Autodesk Inventor part; units mm, degrees
ref_plane "YZ Plane" through (0, 0, 0) normal (1, 0, 0) x (0, 1, 0)
ref_plane "XZ Plane" through (0, 0, 0) normal (0, 1, 0) x (-1, 0, 0)
ref_plane "XY Plane" through (0, 0, 0) normal (0, 0, 1) x (1, 0, 0)
sketch "Sketch1" plane through (0, 0, 0) normal (0, 0, 1) x (1, 0, 0)
  line L0 (0, 0) -> (24, 0)
  line L1 (24, 0) -> (24, 24)
  line L2 (24, 24) -> (0, 24)
  line L3 (0, 24) -> (0, 0)
  dimension "d0" = 24
  dimension "d1" = 24
extrude "Extrusion1" add sketch "Sketch1" along normal blind 15
sketch "Sketch2" plane through (0, 0, 15) normal (0, 0, 1) x (1, 0, 0)
  line L0 (24, 0) -> (24, 24)
  line L1 (24, 24) -> (0, 24)
  line L2 (0, 24) -> (0, 0)
  line L3 (0, 0) -> (24, 0)
  line L4 (2, 22) -> (22, 22)
  line L5 (22, 22) -> (22, 2)
  line L6 (22, 2) -> (2, 2)
  line L7 (2, 2) -> (2, 22)
  dimension "d4" = 2
extrude "Extrusion2" add sketch "Sketch2" along normal blind 2.5
chamfer "Chamfer1" distance 2 angle 45 4 edges at (0, 24, 8.75) (0, 0, 8.75) (24, 0, 8.75) (24, 24, 8.75)
sketch "Sketch3" plane through (0, 0, 0) normal (0, 0, -1) x (-1, 0, 0)
  line L0 (-2, 22) -> (-2, 2)
  line L1 (-2, 2) -> (-22, 2)
  line L2 (-22, 2) -> (-22, 22)
  line L3 (-22, 22) -> (-2, 22)
  point P0 (0, 0)
  point P1 (-12, 16)
  point P2 (-12, 22)
  dimension "d10" = 6
hole "Hole1" at (12, 16, 0) direction (0, 0, 1) diameter 4 depth 24 counterbore diameter 6.5 counterbore depth 10
chamfer "Chamfer2" distance 1 angle 45 8 edges at (12, 0, 0) (23, 1, 0) (24, 12, 0) (23, 23, 0) (12, 24, 0) (0, 12, 0) (1, 23, 0) (1, 1, 0)
thicken "Thicken1" operation add thickness 0.1 both sides no extend neighbours yes toward (1, 0, 0) faces at (22, 15.3333, 16.6667) (15.3333, 2, 16.6667) (2, 8.6667, 16.6667) (8.6667, 22, 15.8333)
chamfer "Chamfer3" distance 1.25 angle 45 1 edges at (12, 14, 10)
properties part number "Idle Side Foot"
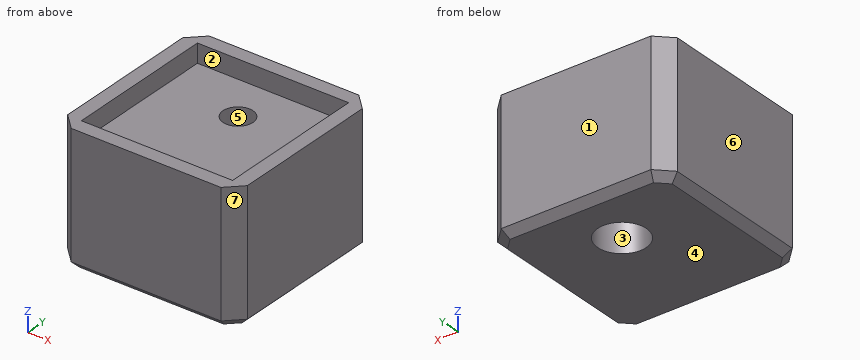
Input: part model. Units: mm. Frame: model coordinates. Face numbers are marked on the shaded views. A direction names the side the tool comes from. Round coordinates to 2 decimals unless told otherwise and drop trailing zeros. Loops run counter-clockwise (first coordinate to the right, second up) from the corner with the lowest first, then second, coordinate; pieces in that order, holes last.
1) Pin query (flat end, axial travel): pin 1 (2 mm diameter, centred on x = 12.5, y = 15.5, fed in from -Z); pin 2 (5 mm diameter, centred on x = 18.5, y = 7.5, fed in from +Z). Return the tip coordinate at first contact, or that it passes through.
Ans:
pin 1: passes through
pin 2: stops at z = 15
2) Set-up query: the marked faces 1, 2 and 3. Return all of +Z, -Z, +X, -X, +Y, -Y with unobstructed straight access to the full face (end or side cutting, diameter ignored); none if empty.
Ans:
face 1: +Z, -Z, +X, -X, +Y
face 2: +Z
face 3: -Z
3) Section query D-D on y = 6.75. Return the cut outline in (x, z).
Ans:
outline: (0, 1) - (1, 0) - (23, 0) - (24, 1) - (24, 17.5) - (22.1, 17.5) - (22.1, 15) - (1.9, 15) - (1.9, 17.5) - (0, 17.5) - close
4) Pull-direction query (X, two-part tool) for the marked faces 4, 5, 6 and 7; classes: released by +X, released by -X, zero draft, split by the parting line, or undercut.
Ans:
face 4: zero draft
face 5: undercut
face 6: released by -X
face 7: released by +X
5) Material intervals for line 1 (X direction, y = 16, z = 5); line 2 (X direction, y = 16, z = 12.15); line 3 (Y direction, x = 12, z = 7.5), sorted ascending.
Ans:
line 1: x = 0 to 8.75, 15.25 to 24
line 2: x = 0 to 10, 14 to 24
line 3: y = 0 to 12.75, 19.25 to 24
6) Section query B-B on z = 3. Return the cut outline in (x, y), plus the area to 3 significant figures.
Ans:
outline: (0, 2) - (2, 0) - (22, 0) - (24, 2) - (24, 22) - (22, 24) - (2, 24) - (0, 22) - close; hole circle Ø6.5 at (12, 16)
area: 535 mm2
